Verification items for the finished model (mm, model axes). Face numbers are marked on the shaded views. Coordinates: 2 decimals unless noted, no trailing zeros. Loops run counter-clockwise (first coordinate to the right, second up) from the corner with the lowest first, then second, coordinate; pieces in that order, holes last. Notation, with made-up numbers: (19, 3.5) -> (73, 3.5) arc R12 ccw to (73, 22.5) -> close; hole circle Ø5 at (-23, -8.75). An arc over 180 degrees is marked (long way). Write item = value, one per line.
```python
from build123d import *

# Parameters (mm, degrees)
BOSS_EXTRUDE1_DEPTH = 304.8
SKETCH2_R           = 9.525
CUT_EXTRUDE1_DEPTH  = 379.664508503


with BuildPart() as part:
    # Sketch1 → Boss-Extrude1 (new body)
    with BuildSketch(Plane.XY):
        Polygon((0, 0), (0, 165.1), (165.1, 165.1), (165.1, 152.4), (12.7, 152.4), (12.7, 0), align=None)
    extrude(amount=BOSS_EXTRUDE1_DEPTH)

    # Sketch2 → Cut-Extrude1 (cut, through all)
    with BuildSketch(Plane.XZ.offset(-152.4)):
        with Locations((88.9, 152.4)):
            Circle(SKETCH2_R)
    extrude(amount=-CUT_EXTRUDE1_DEPTH, mode=Mode.SUBTRACT)


solid = part.part
```
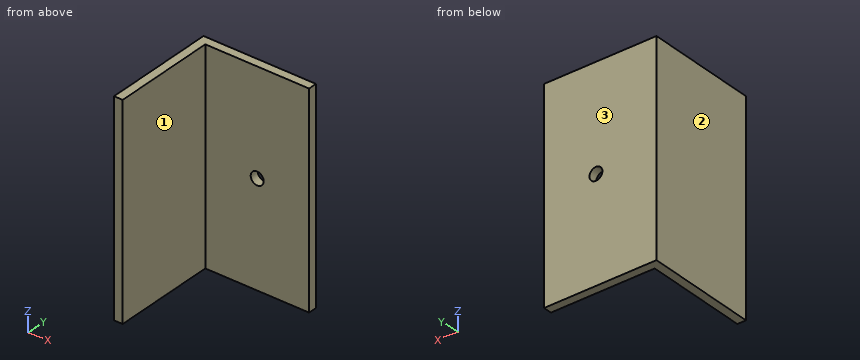
1) Release check for a two-part mould opening along X. For the marked faces 1, 2 and 3 record: pulls with the +X half, pulls with the -X half, needs draft (parallel to the pull), parting line crosses it, or undercut.
Ans:
face_1 = pulls with the +X half
face_2 = pulls with the -X half
face_3 = needs draft
2) Sectioned sample at D-D, the plane x = 134. Record the cut outline in (y, z).
Ans:
outline = (152.4, 0) -> (165.1, 0) -> (165.1, 304.8) -> (152.4, 304.8) -> close
3) Sectioned sample at A-A, the plane z = 152.4. Record the cut outline in (x, y) (3 decimals), plus the area to 3 significant figures.
Ans:
outline = (0, 0) -> (12.7, 0) -> (12.7, 152.4) -> (79.375, 152.4) -> (79.375, 165.1) -> (0, 165.1) -> close; (98.425, 152.4) -> (165.1, 152.4) -> (165.1, 165.1) -> (98.425, 165.1) -> close
area = 3,790 mm2
4) Depth check by flat-ended pin: pin 1 Ø17 at (x, z) = (88.9, 152.4) entering from +Y; pin 2 Ø5 at (x, z) = (125, 100.5) entering from -Y. Enter the tip coordinate at first touch or a pass-through.
Ans:
pin_1 = through
pin_2 = 152.4
5) Sectioned sample at C-C, the plane z = 108.5. Record the cut outline in (x, y), plus the area to 3 significant figures.
Ans:
outline = (0, 0) -> (12.7, 0) -> (12.7, 152.4) -> (165.1, 152.4) -> (165.1, 165.1) -> (0, 165.1) -> close
area = 4,030 mm2
6) Sectioned sample at B-B, the plane x = 88.9. Record the cut outline in (y, z) (3 decimals).
Ans:
outline = (152.4, 0) -> (165.1, 0) -> (165.1, 142.875) -> (152.4, 142.875) -> close; (152.4, 161.925) -> (165.1, 161.925) -> (165.1, 304.8) -> (152.4, 304.8) -> close
7) Material ranges on line 1 (Z direction, x = 88.9, y = 156) (3 decimals); line 2 (X direction, y = 148.5, z = 162); line 3 (Y direction, x = 87.5, z = 292), recorded low to high.
Ans:
line_1 = 0 to 142.875, 161.925 to 304.8
line_2 = 0 to 12.7
line_3 = 152.4 to 165.1
